from build123d import *

# Parameters (mm, degrees)
SKETCH1_R           = 27.325
BOSS_EXTRUDE1_DEPTH = 2.8829
SKETCH2_R           = 25.45715
BOSS_EXTRUDE2_DEPTH = 2.1971
SKETCH6_R           = 6.500596607
CUT_EXTRUDE1_DEPTH  = 25.4


with BuildPart() as part:
    # Sketch1 → Boss-Extrude1 (new body)
    with BuildSketch(Plane(origin=(0, 0, 0), x_dir=(1, 0, 0), z_dir=(0, 1, 0))):
        Circle(SKETCH1_R)
    extrude(amount=BOSS_EXTRUDE1_DEPTH)

    # Sketch2 → Boss-Extrude2 (add)
    with BuildSketch(Plane(origin=(0, 2.8829, 0), x_dir=(1, 0, 0), z_dir=(0, 1, 0))):
        Circle(SKETCH2_R)
    extrude(amount=BOSS_EXTRUDE2_DEPTH)

    # Sketch6 → Cut-Extrude1 (cut)
    with BuildSketch(Plane.XZ):
        Circle(SKETCH6_R)
    extrude(amount=-CUT_EXTRUDE1_DEPTH, mode=Mode.SUBTRACT)


solid = part.part
Read the model definition and answer for the solid it produces. Units are mm, in the model's axes. A direction names the side the tool comes from. Round coordinates to 2 decimals unless told otherwise and drop trailing zeros. Loops run counter-clockwise (first coordinate to the right, second up) from the corner with the lowest first, then second, coordinate; pieces in that order, holes last.
Q1. Section D-D on y = 1.6 is taken. Write down the section's boundary in (x, z) (3 decimals).
Q2. Section B-B on z = 16.5 is taken. Write down the section's boundary in (x, y).
Q3. Each of these flat-tipped pins is pushed along its axis until it touches: pin 1 (1.5 mm diameter, centred on y = 3.5, z = -13, fed in from +X); pin 2 (1.5 mm diameter, centred on x = -10.5, y = 1.5, fed in from +Z); pin 3 (1.5 mm diameter, centred on y = 2, z = 21.5, fed in from -X); pin 4 (12 mm diameter, centred on x = 14.5, z = 4, fed in from -Y). Where does it stop, or does it pass through?
Q4. Consider probe 1 along Z at (x, y) = (0, 4.05); probe 2 along Z at (x, y) = (-6, 2.1); probe 3 along Z at (x, y) = (-11, 4.75). Determine where each line is inside the solid, lowest interval first.
Q5. Section C-C on x = 12 is taken. Write down the section's boundary in (y, z), and give its area (3 significant figures).
Q6. Which of the six approach directions +Z, -Z, +X, -X, +Y, -Y give full straight-line access (tool end or side, diameter ignored) to faces 1 (the face through (-0.846, 2.504, 6.445)), 2 (the face through (24.28, 3.97, -7.65))?
Q7. Section A-A on x = 0 is taken. Write down the section's boundary in (y, z) (3 decimals).
Output:
1. outline: circle Ø54.65 at (0, 0); hole circle Ø13.001 at (0, 0)
2. outline: (-21.78, 0) - (21.78, 0) - (21.78, 2.88) - (19.39, 2.88) - (19.39, 5.08) - (-19.39, 5.08) - (-19.39, 2.88) - (-21.78, 2.88) - close
3. pin 1: stops at x = 24.26
3. pin 2: stops at z = 25.53
3. pin 3: stops at x = -17.78
3. pin 4: stops at y = 0
4. probe 1: z = -25.46 to -6.5, 6.5 to 25.46
4. probe 2: z = -26.66 to -2.5, 2.5 to 26.66
4. probe 3: z = -22.96 to 22.96
5. outline: (0, -24.55) - (2.88, -24.55) - (2.88, -22.45) - (5.08, -22.45) - (5.08, 22.45) - (2.88, 22.45) - (2.88, 24.55) - (0, 24.55) - close
5. area: 240 mm2
6. face 1: +Y, -Y
6. face 2: +Y
7. outline: (0, -27.325) - (2.883, -27.325) - (2.883, -25.457) - (5.08, -25.457) - (5.08, -6.501) - (0, -6.501) - close; (0, 6.501) - (5.08, 6.501) - (5.08, 25.457) - (2.883, 25.457) - (2.883, 27.325) - (0, 27.325) - close
